Input: part model. Units: mm. Frame: model coordinates. A direction names the side the tool comes from. Coordinates: 2 decimals unless noted, no trailing zeros. Order: outer loops, then holes, each group sorted by start corner. A loop starts at its lowest first (then second) coordinate and runs counter-clockwise, first axis right, second up. Notation, with made-up numbers: M -4.5,55.5 L 31.5,55.5 A30 cw 31.5,85.5 Z; hole C 36,-27 d9. An arc over 180 degrees is marked long. Answer in a Markdown table with one row per item.
from build123d import *

# Parameters (mm, degrees)
EXTCUT_DEPTH  = 19.184446463
EXTCUTS_COUNT = 12
EXTCUTS_ANGLE = 330


with BuildPart() as part:
    # SecSke → Base-Revolve (revolve)
    with BuildSketch(Plane.XY, mode=Mode.PRIVATE) as base_revolve_sk:
        Polygon((-4.458387129, 4.616795022), (-7.725510198, 8), (-8.157114079, 7.583204978), (-4.889991009, 4.2), align=None)
    revolve(base_revolve_sk.sketch.rotate(Axis((-34.925, 0, 0), (1, 0, 0)), 90), axis=Axis((-34.925, 0, 0), (1, 0, 0)))

    # ExtCutSke → ExtCut (cut, through all)
    with BuildSketch(Plane(origin=(-7.725510198, 8, 0), x_dir=(0, 0, 1), z_dir=(0.7193398003386475, 0.694658370459001, 0))):
        with BuildLine():
            Line((-0.448786028, 2.297632851), (-1.638758705, -0.238596355))
            ThreePointArc((-1.638758705, -0.238596355), (0, -0.4), (1.638758705, -0.238596355))
            Line((1.638758705, -0.238596355), (0.448786028, 2.297632851))
            ThreePointArc((0.448786028, 2.297632851), (0, 2.28), (-0.448786028, 2.297632851))
        make_face()
    extcut = extrude(amount=-EXTCUT_DEPTH, mode=Mode.SUBTRACT)

    # ExtCuts: ExtCut ×12 about axis
    extcuts_axis = Axis((-34.925, 0, 0), (1, 0, 0))
    for i in range(1, EXTCUTS_COUNT):
        add(extcut.rotate(extcuts_axis, i * EXTCUTS_ANGLE / (EXTCUTS_COUNT - 1)), mode=Mode.SUBTRACT)


solid = part.part
1) Material intervals for probe 1 along Y at (x, z) = (-5.5, 1.75); probe 2 along Y at (x, z) = (-6.5, 4.75); probe 3 along Z at (x, y) = (-6.4, 4), sorted ascending.
Resolved:
| item | result |
|---|---|
| probe 1 | y = -5.42 to -4.5, 4.5 to 5.42 |
| probe 2 | y = -4.77 to -3.44, 3.44 to 4.77 |
| probe 3 | z = -5.28 to -4.15, 4.15 to 5.28 |
2) Cut plane A-A, the plane y = 0. Output: boundary loops of the cut face in (x, z).
Resolved:
| item | result |
|---|---|
| outline | M -6.57,-5.94 L -6.14,-6.36 L -4.46,-4.62 L -4.89,-4.2 Z; M -6.57,5.94 L -4.89,4.2 L -4.46,4.62 L -6.14,6.36 Z |
3) Reachability of faces 1 (the face through (-7.16, 0.97, -6.9)), 2 (the face through (-7.135, 0.957, 6.883)), 3 (the face through (-7.135, 5.482, -4.27)), 4 (the face through (-7.135, -5.482, 4.27)) from +Z, -Z, +X, -X, +Y, -Y: full face, straight path, thin tool, end or side. Return the list, or none.
Resolved:
| item | result |
|---|---|
| face 1 | -Z, -X |
| face 2 | +Z, -X |
| face 3 | -X, +Y |
| face 4 | -X, -Y |
4) Cut plane C-C, the plane x = -7.15. State how many separate pieces and enclosed holes the cut face has, and give its area (3 significant figures).
Resolved:
| item | result |
|---|---|
| separate pieces | 12 |
| enclosed holes | 0 |
| area | 17.7 mm2 |
5) Cut plane D-D, the plane x = -5.9. Output: boundary loops of the cut face in (y, z), and give its area (3 significant figures).
Resolved:
| item | result |
|---|---|
| outline | C 0,0 d12.22; hole C 0,0 d10.49 |
| area | 30.8 mm2 |
6) Contact query for flat-ended pins moving along their axis: pin 1 (2 mm diameter, centred on y = -4, z = -4.5, fed in from +X); pin 2 (1 mm diameter, centred on x = -7.5, z = -5, fed in from +Y). Output: stop coordinate, or through.
Resolved:
| item | result |
|---|---|
| pin 1 | stops at x = -4.85 |
| pin 2 | stops at y = 6.07 |
